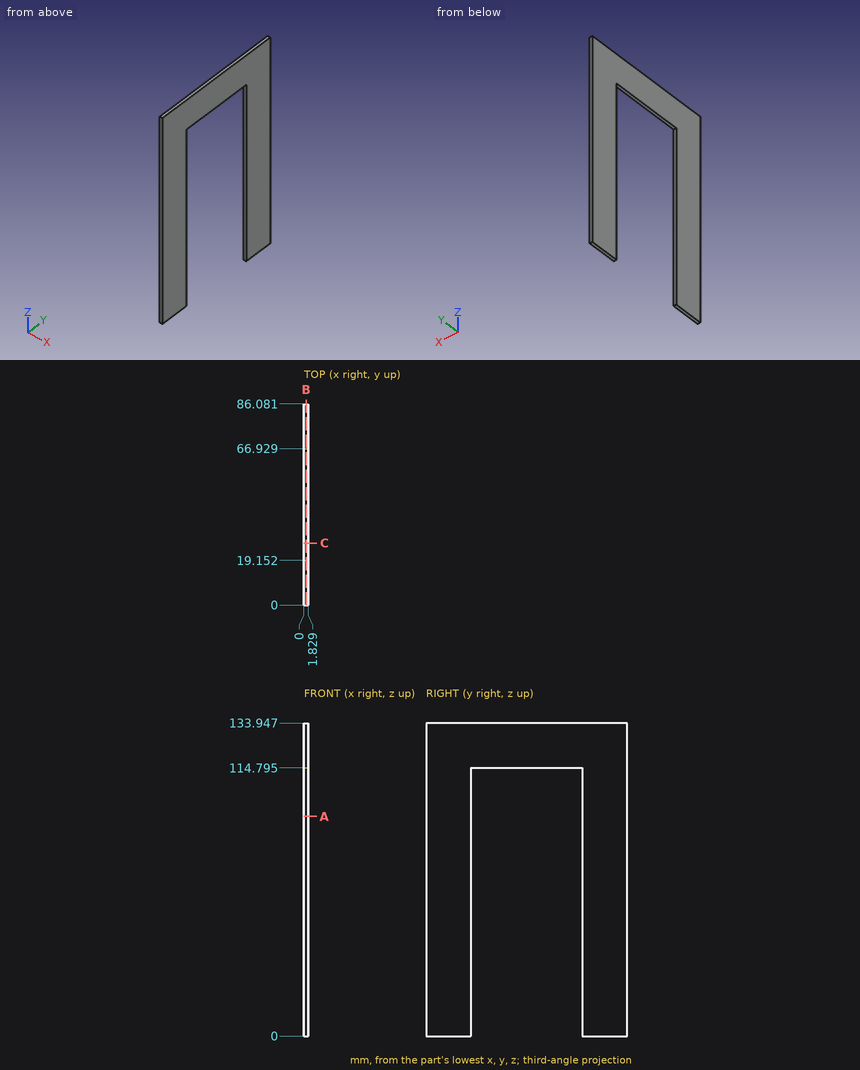
Print and shaded views of the part. All mm, measured from the part's lowest x, y and z. Coordinates: 2 decimals unless noted, no trailing zeros. Order: outer loops, then holes, each group sorted by start corner. A loop starts at its lowest first (then second) coordinate and runs counter-clockwise, first axis right, second up.
(1) Slice it at B-B, the plane x = 0.95. Write the cut outline in (y, z) (1 decimal), and give its area (3 significant figures).
Check sheet entries:
outline: (0, 0) - (19.2, 0) - (19.2, 114.8) - (66.9, 114.8) - (66.9, 0) - (86.1, 0) - (86.1, 133.9) - (0, 133.9) - close
area: 6,050 mm2
(2) Slice it at C-C, the plane y = 26.5. Write the cut outline in (x, z) (1 decimal).
Check sheet entries:
outline: (0, 114.8) - (1.8, 114.8) - (1.8, 133.9) - (0, 133.9) - close
(3) Pin check, flat tip, straight feed: pin 1 Ø0.5 at (x, y) = (0.5, 36.5) entering from -Z (1 decimal). Stop position of the tip, or through.
Check sheet entries:
pin 1: stops at z = 114.8
(4) Probe L1, parallel to Y at x = 0.3, z = 14; L2, parallel to Z at x = 1.45, y = 28.5 (1 decimal). List the from-to ranges inside material, lowest first.
Check sheet entries:
L1: y = 0 to 19.15, 66.93 to 86.08
L2: z = 114.8 to 133.9
(5) Slice it at A-A, the plane z = 94. Write the cut outline in (x, y).
Check sheet entries:
outline: (0, 0) - (1.83, 0) - (1.83, 19.15) - (0, 19.15) - close; (0, 66.93) - (1.83, 66.93) - (1.83, 86.08) - (0, 86.08) - close
